Job drawing, mm, ordinate dimensions from the low corner. One solid piece. A direction names the side the tool comes from. Give positions to 0.01 mm unless a question says otherwise; leave off trailing zeros. Write each loop counter-clockwise with the first axis right and the second up, starting at its lowest first coordinate (ties: lowest second). Pieces come first, ordered by that corner, then holes. Notation, with made-up numbers: (-14, -1) -> (9, -1) arc R30 ccw to (9, 24) -> close; hole circle Ø11 at (44.5, -25). An arc over 180 degrees is marked (long way). Put each result on its own line as item: value. Start each with the question number.
Item 1: Slice it at C-C, the plane y = 28. List the corners of the cut face in (x, z).
Item 2: Drill centre lines: line 1 along Y through (x, z) = (98.5, 20.5) (1 decimal); line 2 along X through (y, z) = (89, 25.5) (1 decimal); line 3 along Z through (x, y) = (106, 80.5). Where is each one in solid material? Low to high.
Item 3: Slice it at B-B, the plane z = 22.5. List the corners of the cut face in (x, y).
Item 4: Tool access for the marked faces 1 and 2: list every direction of +Z, -Z, +X, -X, +Y, -Y with a clear straight run to the whole face (end or side of a thin tool).
Item 5: Slice it at A-A, the plane x = 92.5. List the corners of the cut face in (y, z).
Item 6: Flat gauge pin, fed straight in: pin 1 Ø10.5 at (x, y) = (96.5, 27) entering from -Z. Where does the tip first touch, or does it go through?
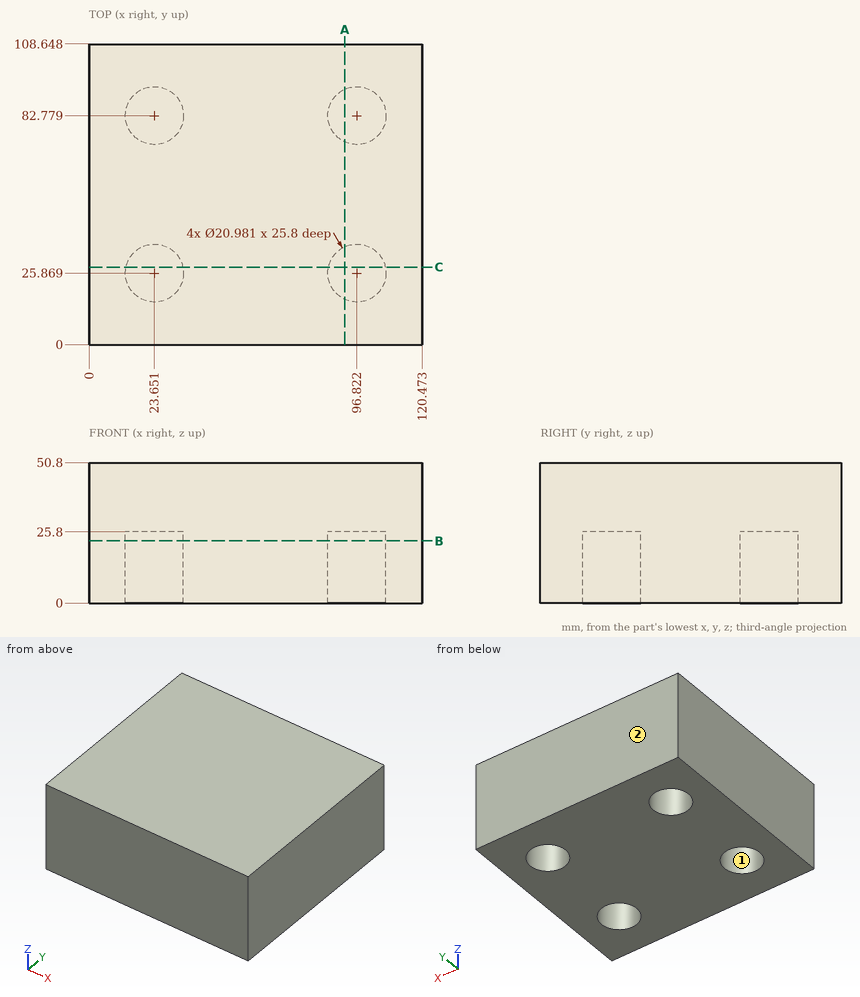
Values follow:
1. outline: (0, 0) -> (13.38, 0) -> (13.38, 25.8) -> (33.92, 25.8) -> (33.92, 0) -> (86.55, 0) -> (86.55, 25.8) -> (107.09, 25.8) -> (107.09, 0) -> (120.47, 0) -> (120.47, 50.8) -> (0, 50.8) -> close
2. line 1: 0 to 15.5, 36.2 to 72.4, 93.1 to 108.6
2. line 2: 0 to 15.2, 32.1 to 88.4, 105.3 to 120.5
2. line 3: 25.8 to 50.8
3. outline: (0, 0) -> (120.47, 0) -> (120.47, 108.65) -> (0, 108.65) -> close; hole circle Ø20.98 at (23.65, 25.87); hole circle Ø20.98 at (23.65, 82.78); hole circle Ø20.98 at (96.82, 25.87); hole circle Ø20.98 at (96.82, 82.78)
4. face 1: -Z
4. face 2: +Z, -Z, +X, -X, +Y
5. outline: (0, 0) -> (16.31, 0) -> (16.31, 25.8) -> (35.43, 25.8) -> (35.43, 0) -> (73.22, 0) -> (73.22, 25.8) -> (92.34, 25.8) -> (92.34, 0) -> (108.65, 0) -> (108.65, 50.8) -> (0, 50.8) -> close
6. pin 1: z = 25.8
